Verification items for the finished model (mm, model axes). A direction names the side the tool comes from. Coordinates: 2 decimals unless noted, no trailing zeros. Order: outer loops, then holes, each group sorted by start corner. A loop starts at its lowest first (then second) coordinate and runs counter-clockwise, first axis right, second up. Notation, with made-up numbers: (-38, 82) -> (4, 82) arc R20 cw to (4, 101) -> close; hole circle Ø11 at (0.25, 65). An arc over 180 degrees is marked (long way). Write item = value, one per line. Start each with the question number.
from build123d import *

# Parameters (mm, degrees)
PAD_DEPTH            = 50
PAD001_DEPTH         = 26.5
PAD001_DEPTH_BACK    = 29
SKETCH001_R          = 3.65
POCKET_DEPTH         = 0.501
POCKET_DEPTH_BACK    = -98.001
SKETCH002_R          = 4
SKETCH002_W          = 9.5
SKETCH002_H          = 30
POCKET001_DEPTH      = 56.001
POCKET001_DEPTH_BACK = -45.501
POCKET002_DEPTH      = 6.5


with BuildPart() as part:
    # Sketch → Pad (new body, symmetric)
    with BuildSketch(Plane.XZ):
        Polygon((-37.5, -28.5), (27, -28.5), (27, 26.5), (43, 26.5), (43, 69.5), (-49.5, 69.5), (-49.5, 26.5), (-37.5, 26.5), align=None)
    extrude(amount=PAD_DEPTH, both=True)

    # Sketch003 → Pad001 (join, two sides)
    with BuildSketch(Plane.XY) as pad001_sk:
        Polygon((-56, -52.5), (-56, -75), (45.5, -75), (45.5, -52.5), (27, -52.5), (27, 52.5), (45.5, 52.5), (45.5, 60), (-56, 60), (-56, 56.5), (-37.5, 56.5), (-37.5, -52.5), align=None)
    extrude(amount=PAD001_DEPTH)
    extrude(pad001_sk.sketch, amount=-PAD001_DEPTH_BACK)

    # Sketch001 → Pocket (cut, two sides)
    with BuildSketch(Plane.XY.offset(-28.5)) as pocket_sk:
        with Locations((0, -7)):
            Circle(SKETCH001_R)
    extrude(amount=-POCKET_DEPTH, mode=Mode.SUBTRACT)
    extrude(pocket_sk.sketch, amount=-POCKET_DEPTH_BACK, mode=Mode.SUBTRACT)

    # Sketch002 → Pocket001 (cut, two sides)
    with BuildSketch(Plane.YZ) as pocket001_sk:
        with Locations((-40, 0)):
            Circle(SKETCH002_R)
        with Locations((40, 0)):
            Circle(SKETCH002_R)
        with Locations((22.75, -15.8)):
            Rectangle(SKETCH002_W, SKETCH002_H)
    extrude(amount=-POCKET001_DEPTH, mode=Mode.SUBTRACT)
    extrude(pocket001_sk.sketch, amount=-POCKET001_DEPTH_BACK, mode=Mode.SUBTRACT)

    # Sketch004 (on DatumPlane) → Pocket002 (cut, symmetric)
    with BuildSketch(Plane(origin=(0.333333, 22.75, -10.033333), x_dir=(-1, 0, 0), z_dir=(0, 1, 0))):
        Polygon((-28.5, 19), (-13.5, 19), (-13.5, 9.2), (-28.5, 9.2), (-28.5, 12), (-18.5, 12), (-18.5, 15), (-28.5, 15), align=None)
        Polygon((38.5, 19), (8.5, 19), (8.5, 9.2), (38.5, 9.2), (38.5, 12), (19.3, 12), (19.3, 15), (38.5, 15), align=None)
    extrude(amount=POCKET002_DEPTH, both=True, mode=Mode.SUBTRACT)


solid = part.part
Item 1: Thickness scan on line 1 (Y direction, x = 0, z = -6); line 2 (Y direction, x = -11, z = 0); line 3 (X direction, y = -7, z = 49). Record the ranges inside material, lowest first.
Item 2: Section check D-D (x = 39). Record the boundary of the cut face in (y, z), then the cut area to 4 significant figures.
Item 3: Tool access check on faces 1 (the flat face through (-47, -52.5, -1)), 2 (the flat face through (-5, 27.5, -15)), 3 (the flat face through (-28, 23, 1.967)), 4 (the flat face through (-6, -62, 26.5)). Record the directions out of +Z, -Z, +X, -X, +Y, -Y that give a thin tool (end or side, any length) a straight path to the whole face; none if there is none.
Item 4: Mould release check, pull along Y, two halves, no side actions. Record for faces 5 (the flat face through (-4, -50, 48)), 6 (the flat face through (-3, -1, 69.5)), 7 (the flat face through (-44, -1, 26.5)): pulls with the +Y half, pulls with the -Y half, needs draft (parallel to the pull), parting line crosses it, or undercut.
Item 5: Section check B-B (x = -16.5). Record the boundary of the cut face in (y, z).
Item 6: Section check A-A (z = -21). Record the boundary of the cut face in (x, y), then the cut area to 3 significant figures.
Item 7: Gauge pin test, flat ends, axial feed: P1, Ø2.5, axis at y = 19.5, z = 3, coming from the -X side; P2, Ø4, axis at x = -24, y = 24, coming from the -Z side; P3, Ø6.5, axis at x = 24, y = 26, coming from the -Z side; P4, Ø8, axis at x = 1, y = 57, coming from the +Z side. Record the tip position at first contact, or that the pin passes through.
Item 8: Section check C-C (z = 20). Record the boundary of the cut face in (x, y), then the cut area to 3 significant figures.
Filled sheet:
q1.line_1 = -75 to -10.65, -3.35 to 18, 27.5 to 60
q1.line_2 = -75 to -44, -36 to 16.25, 29.25 to 36, 44 to 60
q1.line_3 = -49.5 to -3.65, 3.65 to 43
q2.outline = (-75, -29) -> (-52.5, -29) -> (-52.5, 26.5) -> (-75, 26.5) -> close; (-50, 26.5) -> (50, 26.5) -> (50, 69.5) -> (-50, 69.5) -> close; (52.5, -29) -> (60, -29) -> (60, 26.5) -> (52.5, 26.5) -> close
q2.area = 5,965 mm^2
q3.face_1 = +Z, -Z, -X
q3.face_2 = -Z, +X, -X
q3.face_3 = -X
q3.face_4 = +Z, +X, -X, -Y
q4.face_5 = pulls with the -Y half
q4.face_6 = needs draft
q4.face_7 = undercut
q5.outline = (-75, -29) -> (18, -29) -> (18, -0.83) -> (16.25, -0.83) -> (16.25, 8.97) -> (29.25, 8.97) -> (29.25, -0.83) -> (27.5, -0.83) -> (27.5, -29) -> (60, -29) -> (60, 26.5) -> (50, 26.5) -> (50, 69.5) -> (-50, 69.5) -> (-50, 26.5) -> (-75, 26.5) -> close; hole circle Ø8 at (-40, 0); hole circle Ø8 at (40, 0)
q6.outline = (-56, -75) -> (45.5, -75) -> (45.5, -52.5) -> (27, -52.5) -> (27, 18) -> (-37.5, 18) -> (-37.5, -52.5) -> (-56, -52.5) -> close; (-56, 56.5) -> (-37.5, 56.5) -> (-37.5, 27.5) -> (27, 27.5) -> (27, 52.5) -> (45.5, 52.5) -> (45.5, 60) -> (-56, 60) -> close; hole circle Ø7.3 at (0, -7)
q6.area = 9,090 mm^2
q7.P1 = -37.5
q7.P2 = 1.97
q7.P3 = -29
q7.P4 = 26.5
q8.outline = (-56, -75) -> (45.5, -75) -> (45.5, -52.5) -> (27, -52.5) -> (27, 52.5) -> (45.5, 52.5) -> (45.5, 60) -> (-56, 60) -> (-56, 56.5) -> (-37.5, 56.5) -> (-37.5, -52.5) -> (-56, -52.5) -> close; hole circle Ø7.3 at (0, -7)
q8.area = 9,700 mm^2
